CAD build for the part. Positions are in the model's coordinates, mm. A direction names the side the tool comes from. Give positions to 0.01 mm unless a question says otherwise; leave off trailing zeros. Put each result on its own line as item: value. Start each with the question number.
1. Cut at A-A on z = 351.5. Give the number of separate pieces and of enclosed holes in the cut face, and give its area (3 significant figures).
2. Tool access for faces 1 (the flat face through (0, -7.75, 246)), 2 (the flat face through (20, -10, 246)): list every direction of +Z, -Z, +X, -X, +Y, -Y with a clear straight run to the whole face (end or side of a thin tool).
3. Drop flat-ended pins along their axis: pin 1 (0.8 mm diameter, centred on y = 17, z = 276, fed in from +X); pin 2 (0.8 mm diameter, centred on x = -16.5, z = 134.5, fed in from -Y); pin 3 (4 mm diameter, centred on x = -3, y = -12.5, fed in from +Z); pin 4 (4 mm diameter, centred on y = 0, z = 148, fed in from +X). Give the stop position or say it passes through.
4. Wall check: line 1 (Y direction, x = -5.5, z = 87.5); line 2 (X direction, y = -13, z = 122.5). Give the ranges that are in metal, low to high.
from build123d import *

# Parameters (mm, degrees)
SKETCH1_R           = 3.4
BOSS_EXTRUDE1_DEPTH = 500


with BuildPart() as part:
    # Sketch1 → Boss-Extrude1 (new body)
    with BuildSketch(Plane.XY):
        with BuildLine():
            Line((7.75, -6.335786438), (7.75, 6.335786438))
            Line((7.75, 6.335786438), (11.664213562, 10.25))
            Line((11.664213562, 10.25), (18, 10.25))
            Line((18, 10.25), (18, 6.1))
            Line((18, 6.1), (15.5, 6.1))
            Line((15.5, 6.1), (15.5, 4.1))
            Line((15.5, 4.1), (20, 4.1))
            Line((20, 4.1), (20, 15.5))
            ThreePointArc((20, 15.5), (18.681980515, 18.681980515), (15.5, 20))
            Line((15.5, 20), (4.1, 20))
            Line((4.1, 20), (4.1, 15.5))
            Line((4.1, 15.5), (6.1, 15.5))
            Line((6.1, 15.5), (6.1, 18))
            Line((6.1, 18), (10.25, 18))
            Line((10.25, 18), (10.25, 11.664213562))
            Line((10.25, 11.664213562), (6.335786438, 7.75))
            Line((6.335786438, 7.75), (-6.335786438, 7.75))
            Line((-6.335786438, 7.75), (-10.25, 11.664213562))
            Line((-10.25, 11.664213562), (-10.25, 18))
            Line((-10.25, 18), (-6.1, 18))
            Line((-6.1, 18), (-6.1, 15.5))
            Line((-6.1, 15.5), (-4.1, 15.5))
            Line((-4.1, 15.5), (-4.1, 20))
            Line((-4.1, 20), (-15.5, 20))
            ThreePointArc((-15.5, 20), (-18.681980515, 18.681980515), (-20, 15.5))
            Line((-20, 15.5), (-20, 4.1))
            Line((-20, 4.1), (-15.5, 4.1))
            Line((-15.5, 4.1), (-15.5, 6.1))
            Line((-15.5, 6.1), (-18, 6.1))
            Line((-18, 6.1), (-18, 10.25))
            Line((-18, 10.25), (-11.664213562, 10.25))
            Line((-11.664213562, 10.25), (-7.75, 6.335786438))
            Line((-7.75, 6.335786438), (-7.75, -6.335786438))
            Line((-7.75, -6.335786438), (-11.664213562, -10.25))
            Line((-11.664213562, -10.25), (-18, -10.25))
            Line((-18, -10.25), (-18, -6.1))
            Line((-18, -6.1), (-15.5, -6.1))
            Line((-15.5, -6.1), (-15.5, -4.1))
            Line((-15.5, -4.1), (-20, -4.1))
            Line((-20, -4.1), (-20, -15.5))
            ThreePointArc((-20, -15.5), (-18.681980515, -18.681980515), (-15.5, -20))
            Line((-15.5, -20), (-4.1, -20))
            Line((-4.1, -20), (-4.1, -15.5))
            Line((-4.1, -15.5), (-6.1, -15.5))
            Line((-6.1, -15.5), (-6.1, -18))
            Line((-6.1, -18), (-10.25, -18))
            Line((-10.25, -18), (-10.25, -11.664213562))
            Line((-10.25, -11.664213562), (-6.335786438, -7.75))
            Line((-6.335786438, -7.75), (6.335786438, -7.75))
            Line((6.335786438, -7.75), (10.25, -11.664213562))
            Line((10.25, -11.664213562), (10.25, -18))
            Line((10.25, -18), (6.1, -18))
            Line((6.1, -18), (6.1, -15.5))
            Line((6.1, -15.5), (4.1, -15.5))
            Line((4.1, -15.5), (4.1, -20))
            Line((4.1, -20), (15.5, -20))
            ThreePointArc((15.5, -20), (18.681980515, -18.681980515), (20, -15.5))
            Line((20, -15.5), (20, -4.1))
            Line((20, -4.1), (15.5, -4.1))
            Line((15.5, -4.1), (15.5, -6.1))
            Line((15.5, -6.1), (18, -6.1))
            Line((18, -6.1), (18, -10.25))
            Line((18, -10.25), (11.664213562, -10.25))
            Line((11.664213562, -10.25), (7.75, -6.335786438))
        make_face()
        Circle(SKETCH1_R, mode=Mode.SUBTRACT)
        with BuildLine():
            Line((15.5, 18), (12.25, 18))
            Line((12.25, 18), (12.25, 12.25))
            Line((12.25, 12.25), (18, 12.25))
            Line((18, 12.25), (18, 15.5))
            ThreePointArc((18, 15.5), (17.267766953, 17.267766953), (15.5, 18))
        make_face(mode=Mode.SUBTRACT)
        with BuildLine():
            Line((-15.5, 18), (-12.25, 18))
            Line((-12.25, 18), (-12.25, 12.25))
            Line((-12.25, 12.25), (-18, 12.25))
            Line((-18, 12.25), (-18, 15.5))
            ThreePointArc((-18, 15.5), (-17.267766953, 17.267766953), (-15.5, 18))
        make_face(mode=Mode.SUBTRACT)
        with BuildLine():
            Line((-15.5, -18), (-12.25, -18))
            Line((-12.25, -18), (-12.25, -12.25))
            Line((-12.25, -12.25), (-18, -12.25))
            Line((-18, -12.25), (-18, -15.5))
            ThreePointArc((-18, -15.5), (-17.267766953, -17.267766953), (-15.5, -18))
        make_face(mode=Mode.SUBTRACT)
        with BuildLine():
            Line((15.5, -18), (12.25, -18))
            Line((12.25, -18), (12.25, -12.25))
            Line((12.25, -12.25), (18, -12.25))
            Line((18, -12.25), (18, -15.5))
            ThreePointArc((18, -15.5), (17.267766953, -17.267766953), (15.5, -18))
        make_face(mode=Mode.SUBTRACT)
    extrude(amount=BOSS_EXTRUDE1_DEPTH)


solid = part.part
Report:
1. separate pieces: 1
1. enclosed holes: 5
1. area: 615 mm²
2. face 1: +Z, -Z
2. face 2: +Z, -Z, +X, +Y, -Y
3. pin 1: stops at x = 19.86
3. pin 2: stops at y = -19.96
3. pin 3: passes through
3. pin 4: stops at x = 7.75
4. line 1: y = -20 to -15.5, -7.75 to 7.75, 15.5 to 20
4. line 2: x = -20 to -18, -12.25 to -10.25, 10.25 to 12.25, 18 to 20
